Geometry: see drawing. Coordinates: mm, zero at the bounding-box minimum. Give positions to 0.01 mm unless a question says otherwise; leave off trailing zeros. Loops run counter-clockwise (first coordinate to the right, second up) from the corner with the lowest first, then second, coordinate; pieces in that order, holes last. Notation, with made-up numbers: (14.25, 77.25) -> (61.25, 77.25) arc R31 cw to (61.25, 111.25) -> close; hole circle Ø8 at (-23, -19.75). An arc over 180 degrees is marked (long way). Use CSV: the item, a comma, the result in double quotes.
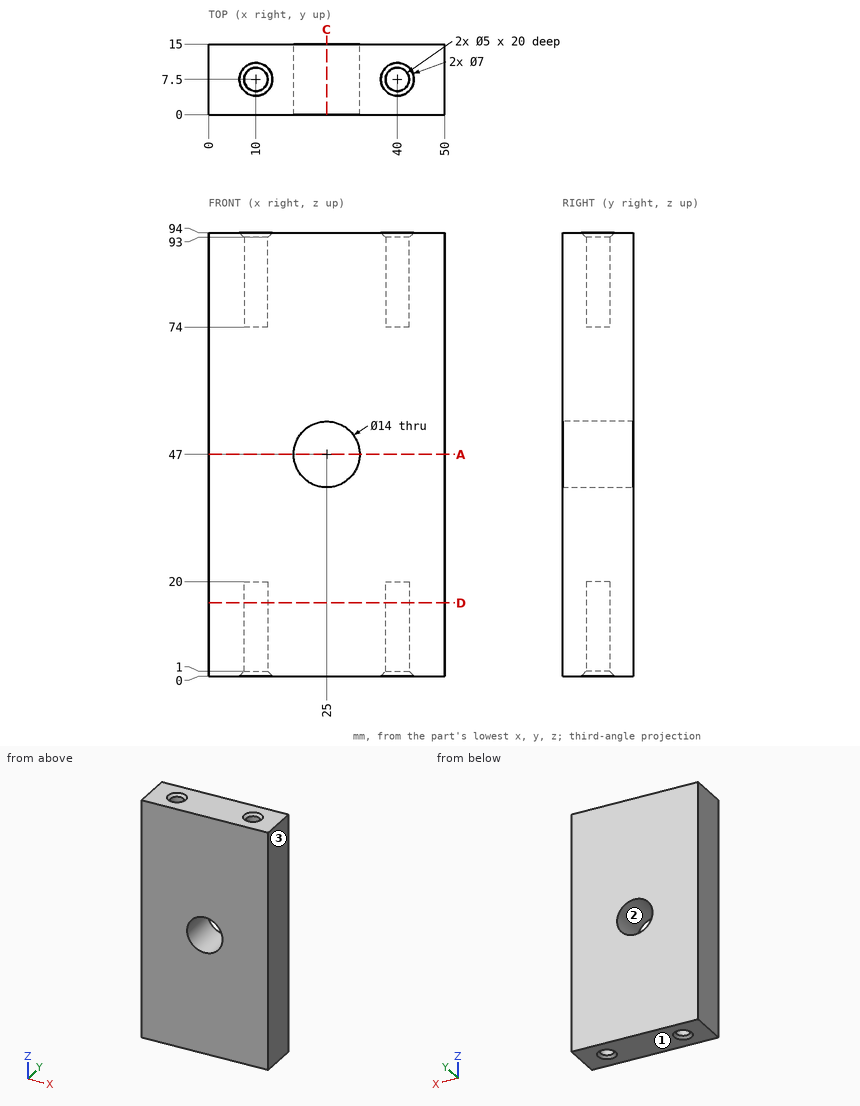
1) Ray query, line 1 (Y direction, x = 40, z = 85); line 2 (X direction, y = 7, z = 89.5); line 3 (X direction, y = 9.5, z = 47). Return the intervals inside material, ascending.
From the geometry:
line 1,"y = 0 to 5, 10 to 15"
line 2,"x = 0 to 7.55, 12.45 to 37.55, 42.45 to 50"
line 3,"x = 0 to 18, 32 to 50"
2) Section query A-A (z = 47). Return loops of the section in (x, y), then the cut area to 3 significant figures.
From the geometry:
outline,"(0, 0) -> (18, 0) -> (18, 15) -> (0, 15) -> close; (32, 0) -> (50, 0) -> (50, 15) -> (32, 15) -> close"
area,"540 mm^2"
3) Section query C-C (x = 25). Return loops of the section in (y, z).
From the geometry:
outline,"(0, 0) -> (15, 0) -> (15, 40) -> (0, 40) -> close; (0, 54) -> (15, 54) -> (15, 94) -> (0, 94) -> close"
4) Contact query for flat-ended pins moving along their axis: pin 1 (6 mm diameter, centred on x = 40, y = 7.5, fed in from +Z); pin 2 (1.5 mm diameter, centred on x = 11, y = 8, fed in from +Z); pin 3 (1.5 mm diameter, centred on x = 11, y = 7, fed in from -Z). Output: stop coordinate, or through.
From the geometry:
pin 1,"stops at z = 93.5"
pin 2,"stops at z = 74"
pin 3,"stops at z = 20"
5) Section query D-D (z = 15.5). Return loops of the section in (x, y), then the cut area to 3 significant figures.
From the geometry:
outline,"(0, 0) -> (50, 0) -> (50, 15) -> (0, 15) -> close; hole circle Ø5 at (10, 7.5); hole circle Ø5 at (40, 7.5)"
area,"711 mm^2"
6) Mould query, pull axis Z, two halves, no side actions, for the marked faces 1, 2 and 3. Classes: pulls with the +Z half, pulls with the -Z half, needs draft (parallel to the pull), parting line crosses it, or undercut.
From the geometry:
face 1,"pulls with the -Z half"
face 2,"undercut"
face 3,"needs draft"
